Work out the finished part from the listing and answer in its coordinate system (mm). A direction names the side the tool comes from. Coordinates: 2 decimals unless noted, no trailing zeros. Order: outer loops, then holes, each group sorted by start corner. A loop starts at its lowest first (then second) coordinate and runs counter-clockwise, first axis right, second up. Notation, with made-up numbers: (59.25, 71) - (112.25, 71) arc R8 ccw to (112.25, 86) - close; hole circle Ø11 at (89.5, 30). An arc over 180 degrees is marked (long way). Answer as a JSON object with one key per item and string values. Group by question number.
1) The mould has two halves that part along X. Classify faces 4 (the face through (3.393, 3.397, -1.11)), 5 (the face through (0, 3, -3.57)), 6 (the face through (-2, 0, 2)), 7 (the face through (1.6, 0.2, 0)): released by +X, released by -X, zero draft, split by the parting line, or undercut.
2) Section D-D (z = -3) is taken. Give the vertices of the cut face in (x, y), plus the area to 3 significant figures.
3) Section C-C (z = -4) is taken. Give the vertices of the cut face in (x, y), plus the area to 3 significant figures.
4) Section B-B (x = 0) is taken. Give the vertices of the cut face in (y, z), plus the area to 3 significant figures.
5) Each of these flat-tipped pins is pushed along its axis until it touches: P1, Ø3, axis at y = 3, z = 2.5, coming from the -X side; P2, Ø0.8, axis at x = 0, y = 3.5, coming from the -Z side; P3, Ø0.9, axis at x = 1.5, z = 0.5, coming from the +Y side. Where does it stop, or does it pass through?
6) Find the intervals of material crossed by line 1 along Z through (x, y) = (0, 1.75); line 2 along X through (y, z) = (2.5, 0); line 3 along Z through (x, y) = (3.75, 1.5), in increasing order.
7) Section A-A (z = 0) is taken. Give the vertices of the cut face in (x, y).
8) A tool of negligible diameter and unlimited length cuts with its end or side. For faces 1 (the face through (0, 3, 3.57)), 2 (the face through (-3.397, 3.397, -1.097)), 3 (the face through (1.4, 3, 0)), from which of +Z, -Z, +X, -X, +Y, -Y can it reach the whole face along a straight path? Write none if from no direction.
from build123d import *

# Parameters (mm, degrees)
SKIZZE1_R                       = 4.57
SKIZZE1_R_2                     = 2
AUFSATZ_LINEAR_AUSTRAGEN1_DEPTH = 6.7
SCHNITT_LINEAR_AUSTRAGEN1_DEPTH = 7.7
VERRUNDUNG1_R                   = 0.5
KREISMUSTER1_COUNT              = 10
VERRUNDUNG1_OF_KREISMUSTER1_R   = 0.5
FASE2_SIZE                      = 0.2
BOSS_EXTRUDE1_DEPTH             = 3.15
BOSS_EXTRUDE1_DEPTH_BACK        = 3.15
FILLET1_R                       = 0.5


with BuildPart() as part:
    # Skizze1 → Aufsatz-Linear austragen1 (new body)
    with BuildSketch(Plane(origin=(0, 0, 0), x_dir=(1, 0, 0), z_dir=(0, 1, 0))):
        Circle(SKIZZE1_R)
        Circle(SKIZZE1_R_2, mode=Mode.SUBTRACT)
    extrude(amount=AUFSATZ_LINEAR_AUSTRAGEN1_DEPTH)

    # Skizze12 → Schnitt-Linear austragen1 (cut, through all)
    with BuildSketch(Plane(origin=(0, 6.7, 0), x_dir=(1, 0, 0), z_dir=(0, 1, 0))):
        with BuildLine():
            Line((-1.2, 4.409637173), (-0.808470756, 3.57))
            Line((-0.808470756, 3.57), (0.808470756, 3.57))
            Line((0.808470756, 3.57), (1.2, 4.409637173))
            ThreePointArc((1.2, 4.409637173), (0, 4.57), (-1.2, 4.409637173))
        make_face()
    schnitt_linear_austragen1 = extrude(amount=-SCHNITT_LINEAR_AUSTRAGEN1_DEPTH, mode=Mode.SUBTRACT)

    # Verrundung1
    verrundung1_edges = [part.edges().sort_by_distance(p)[0] for p in [
        (0.808470756, 3.35, -3.57),
        (-0.808470756, 3.35, -3.57),
    ]]
    fillet(verrundung1_edges, radius=VERRUNDUNG1_R)

    # Kreismuster1: Schnitt-Linear austragen1 ×10 about axis
    kreismuster1_axis = Axis((0, 0, 0), (0, 1, 0))
    for i in range(1, KREISMUSTER1_COUNT):
        add(schnitt_linear_austragen1.rotate(kreismuster1_axis, i * 360 / KREISMUSTER1_COUNT), mode=Mode.SUBTRACT)

    # Verrundung1 of Kreismuster1
    verrundung1_of_kreismuster1_edges = [part.edges().sort_by_distance(p)[0] for p in [
        (-1.44432677, 3.35, -3.363397857),
        (-2.752459932, 3.35, -2.412983483),
        (-3.14544056, 3.35, -1.872092051),
        (-3.645102966, 3.35, -0.334289289),
        (-3.645102966, 3.35, 0.334289289),
        (-3.14544056, 3.35, 1.872092051),
        (-2.752459932, 3.35, 2.412983483),
        (-1.44432677, 3.35, 3.363397857),
        (-0.808470756, 3.35, 3.57),
        (0.808470756, 3.35, 3.57),
        (1.44432677, 3.35, 3.363397857),
        (2.752459932, 3.35, 2.412983483),
        (3.14544056, 3.35, 1.872092051),
        (3.645102966, 3.35, 0.334289289),
        (3.645102966, 3.35, -0.334289289),
        (3.14544056, 3.35, -1.872092051),
        (2.752459932, 3.35, -2.412983483),
        (1.44432677, 3.35, -3.363397857),
    ]]
    fillet(verrundung1_of_kreismuster1_edges, radius=VERRUNDUNG1_OF_KREISMUSTER1_R)

    # Fase2
    fase2_edges = [part.edges().sort_by_distance(p)[0] for p in [
        (-2, 0, 0),
        (-2, 6.7, 0),
    ]]
    chamfer(fase2_edges, length=FASE2_SIZE)

    # Sketch1 → Boss-Extrude1 (add, two sides)
    with BuildSketch(Plane(origin=(0, 3.35, 0), x_dir=(-1, 0, 0), z_dir=(0, -1, 0))) as boss_extrude1_sk:
        with BuildLine():
            Line((-1.4, 1.428285686), (-1.4, -1.428285686))
            ThreePointArc((-1.4, -1.428285686), (-2, 0), (-1.4, 1.428285686))
        make_face()
    extrude(amount=BOSS_EXTRUDE1_DEPTH)
    extrude(boss_extrude1_sk.sketch, amount=-BOSS_EXTRUDE1_DEPTH_BACK)

    # Fillet1
    fillet1_edges = [part.edges().sort_by_distance(p)[0] for p in [
        (1.4, 3.35, 1.428285686),
        (1.4, 3.35, -1.428285686),
    ]]
    fillet(fillet1_edges, radius=FILLET1_R)


solid = part.part
Report:
{
 "1": {"face 4": "released by +X", "face 5": "undercut", "face 6": "zero draft", "face 7": "undercut"},
 "2": {"outline": "(-1.94, 0) - (1.94, 0) - (1.94, 6.7) - (-1.94, 6.7) - close", "area": "26.1 mm²"},
 "3": {"outline": "(-1.57, 0) - (-1.01, 0) - (-1.01, 6.7) - (-1.57, 6.7) - close; (1.01, 0) - (1.57, 0) - (1.57, 6.7) - (1.01, 6.7) - close", "area": "7.49 mm²"},
 "4": {"outline": "(0, -3.57) - (6.7, -3.57) - (6.7, -2.2) - (6.5, -2) - (0.2, -2) - (0, -2.2) - close; (0, 2.2) - (0.2, 2) - (6.5, 2) - (6.7, 2.2) - (6.7, 3.57) - (0, 3.57) - close", "area": "21.0 mm²"},
 "5": {"P1": "stops at x = -3.82", "P2": "stops at z = -3.57", "P3": "stops at y = 6.53"},
 "6": {"line 1": "z = -3.57 to -2, 2 to 3.57", "line 2": "x = -4.57 to -2, 1.4 to 4.57", "line 3": "z = -2.61 to -2.44, -0.37 to 0.37, 2.44 to 2.61"},
 "7": {"outline": "(-4.57, 0) - (-2.2, 0) - (-2, 0.2) - (-2, 6.5) - (-2.2, 6.7) - (-4.57, 6.7) - close; (1.4, 0.2) - (2, 0.2) - (2.2, 0) - (4.57, 0) - (4.57, 6.7) - (2.2, 6.7) - (2, 6.5) - (1.4, 6.5) - close"},
 "8": {"face 1": "+Z, +Y, -Y", "face 2": "-X, +Y, -Y", "face 3": "+Y, -Y"}
}
